Can you work these out from the model? Positions are in its coordinate system, mm. A direction names the side the tool comes from. Give positions to 0.01 mm unless a question says otherwise; leave off trailing zeros. Order: outer loops, then holes, each group sorted by start corner. A loop starts at its lowest first (then second) coordinate and runs counter-clockwise, first axis right, second up. Notation, with made-up numbers: M 26.25,18.5 L 43.25,18.5 A13 cw 43.25,31.5 Z; hole C 0.5,-33 d6. An arc over 180 degrees is marked long. One line per question, with ' | ' between items. Start each with the question number.
1) If we section it at A-A, the plane y = -8.5: Please give me the cut outline in (x, z).
2) Please list where these lines run through material, in increasing order: line 1 along Z through (x, y) = (2.5, 0); line 2 along Y through (x, z) = (-3.75, -0.5); line 3 along X through (y, z) = (0.75, 5.5). Write a range as [from, to].
3) If we section it at B-B, the plane x = -4: Please give me the cut outline in (y, z), plus the area to 3 significant figures.
4) If we section it at D-D, the plane y = 0: Please give me the cut outline in (x, z).
5) Thinking about a two-plate mould opening in Z: for faces 1 (the cylindrical face through (-0.9, -7, -0.9)), 2 (the flat face through (0, -5, 0)), 3 (the conical face through (-4.865, 12.135, -0.124)), which applies, +Z half, -Z half, draft (parallel to the pull), parting line (faces both ways), or undercut?
6) For faces 4 (the cylindrical face through (5.3, -1.08, -4.88)), 5 (the flat face through (-1.9, -10.5, 0)), 6 (the cylindrical face through (0.789, 2.192, -4.214)), which set-ups out of +Z, -Z, +X, -X, +Y, -Y let a thin tool reach every point of the face, with its end or its side?
7) I'm going to push flat-ended pins straight in: pin 1 Ø1 at (x, y) = (3.5, 2) entering from +Z; pin 2 Ø2 at (x, z) = (1.5, -5) entering from -Y; pin 3 Ø3 at (y, z) = (-8.5, 0) entering from -X; pin 4 Ø5.5 at (y, z) = (8.5, 0) entering from -X. Where does each tip first touch, or does it pass through?
8) If we section it at C-C, the plane z = 0: State how many separate pieces and enclosed holes the cut face has, plus the area to 3 significant figures.
```python
from build123d import *

# Parameters (mm, degrees)
CHAMFER1_SIZE          = 0.5
FILLET1_R              = 0.9
CUT_EXTRUDE2_DEPTH     = 6
CAP_SCREW2_D           = 3.5
CAP_SCREW2_CBORE_D     = 6
CAP_SCREW2_CBORE_DEPTH = 3.1


with BuildPart() as part:
    # Sketch1 → Revolve1 (revolve)
    with BuildSketch(Plane.XY):
        Polygon((-5, 2.5), (10, 2.5), (10, 5), (1.6, 5), (1.6, 4.75), (0, 4.75), (0, 12.5), (-5, 12.5), align=None)
    revolve(axis=Axis((-5, 0, 0), (1, 0, 0)))

    # Chamfer1
    chamfer1_edges = [part.edges().sort_by_distance(p)[0] for p in [
        (0, -12.5, 0),
        (-5, -12.5, 0),
    ]]
    chamfer(chamfer1_edges, length=CHAMFER1_SIZE)

    # Fillet1
    fillet1_edges = [part.edges().sort_by_distance(p)[0] for p in [
        (10, -5, 0),
    ]]
    fillet(fillet1_edges, radius=FILLET1_R)

    # Sketch5 → Cut-Extrude2 (cut, through all)
    with BuildSketch(Plane.ZY):
        with BuildLine():
            Line((-8, 9.604686356), (-8, -9.604686356))
            ThreePointArc((-8, -9.604686356), (-12.5, 0), (-8, 9.604686356))
        make_face()
        with BuildLine():
            Line((8, 9.604686356), (8, -9.604686356))
            ThreePointArc((8, -9.604686356), (12.5, 0), (8, 9.604686356))
        make_face()
    extrude(amount=CUT_EXTRUDE2_DEPTH, mode=Mode.SUBTRACT)

    # Cap Screw2 (through all)
    with Locations(Plane.ZY.offset(5)):
        with Locations((0, -8.5), (0, 8.5)):
            CounterBoreHole(CAP_SCREW2_D / 2, CAP_SCREW2_CBORE_D / 2, CAP_SCREW2_CBORE_DEPTH)


solid = part.part
```
Results found:
1) outline: M -5,-8 L 0,-8 L 0,-1.75 L -1.9,-1.75 L -1.9,-3 L -5,-3 Z; M -5,3 L -1.9,3 L -1.9,1.75 L 0,1.75 L 0,8 L -5,8 Z
2) line 1: z = [-5, -2.5], [2.5, 5] | line 2: y = [-12.49, -11.46], [-5.54, -2.45], [2.45, 5.54], [11.46, 12.49] | line 3: x = [-5, 0]
3) outline: M -9.6,-8 L 9.6,-8 A12.5 ccw 9.6,8 L -9.6,8 A12.5 ccw Z; hole C -8.5,0 d6; hole C 0,0 d5; hole C 8.5,0 d6 | area: 295 mm²
4) outline: M -5,-8 L 0,-8 L 0,-4.75 L 1.6,-4.75 L 1.6,-5 L 9.1,-5 A0.9 ccw 10,-4.1 L 10,-2.5 L -5,-2.5 Z; M -5,2.5 L 10,2.5 L 10,4.1 A0.9 ccw 9.1,5 L 1.6,5 L 1.6,4.75 L 0,4.75 L 0,8 L -5,8 Z
5) face 1: undercut | face 2: draft | face 3: parting line
6) face 4: +X | face 5: -X | face 6: none
7) pin 1: stops at z = 4.77 | pin 2: stops at y = -2.99 | pin 3: passes through | pin 4: stops at x = -1.9
8) separate pieces: 4 | enclosed holes: 0 | area: 97.9 mm²
